from build123d import *

# Parameters (mm, degrees)
F1_DEPTH = 15
F2_DEPTH = 83.82


with BuildPart() as f1:
    # F0 (on Top) → F1 (new body, symmetric)
    with BuildSketch(Plane.XY):
        Polygon((20.593876, 37.709061), (-42.857531, 35.482697), (-40.909462, 15.167112), (-40.909462, -7.65313), (-11.131826, -49.954068), (28.386155, -49.954068), (38.404796, -35.482697), (0.953089, -31.724066), (0, -19.619845), (35.34355, -16.836887), (32.003999, 0), (13.142763, 16.280918), (28.107863, 25.464052), align=None)
    extrude(amount=F1_DEPTH, both=True)

    # F1_face (on face) → F2 (join)
    with BuildSketch(Plane(origin=(-4.856756, -2.869367, 15), x_dir=(1, 0, 0), z_dir=(0, 0, 1))):
        Polygon((5.809844, -28.854699), (4.856756, -16.750478), (40.200306, -13.96752), (36.860755, 2.869367), (17.999519, 19.150285), (32.964619, 28.333419), (25.450632, 40.578428), (-38.000776, 38.352064), (-36.052706, 18.036479), (-36.052706, -4.783763), (-6.27507, -47.084701), (33.242911, -47.084701), (43.261552, -32.61333), align=None)
    extrude(amount=F2_DEPTH)


solid = f1.part
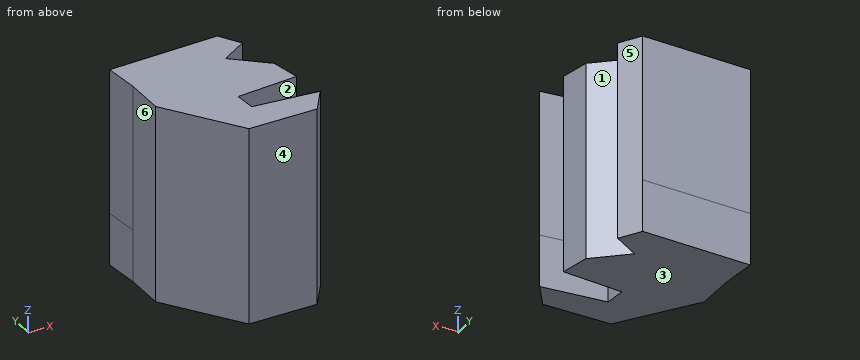
The listing builds one solid part. Answer for the finished solid, in the listing's coordinates (mm). Face numbers are marked on the shaded views. A direction names the side the tool comes from. Coordinates: 2 decimals unless noted, no trailing zeros. Order: outer loops, then holes, each group sorted by start corner. A loop starts at its lowest first (then second) coordinate and runs counter-clockwise, first axis right, second up.
Q1. A cutting plane is placed at D-D, the plane x = -38. Write down the section's boundary in (y, z).
Q2. A cutting plane is placed at A-A, the plane x = 3. Write down the section's boundary in (y, z), and give its area (3 significant figures).
Q3. A cutting plane is placed at B-B, the plane z = 90. Write down the section's boundary in (x, y).
Q4. Consider line 1 (Y direction, x = 15, z = 34); line 2 (Y direction, x = 14, z = 5.5); line 3 (Y direction, x = 12.5, z = 60.5). Determine where each line is inside the solid, lowest interval first.
Q5. For a pull along Y with two mould halves and no side action, classify the marked faces 1, 2, 3 and 4 as pulls with the +Y half, pulls with the -Y half, needs draft (parallel to the pull), parting line crosses it, or undercut.
Q6. Which of the six approach directions +Z, -Z, +X, -X, +Y, -Y give full straight-line access (tool end or side, diameter ignored) to the marked faces 5 and 6?
Q7. Given P1, Ø2, axis at y = -22, z = 61.5, coming from the -X side; P2, Ø5, axis at y = 23, z = 34.5, coming from the +X side; P3, Ø18.5, axis at y = 3, z = 62, coming from the -X side, each flat-ended and moving along its own axis, determine where each tip first touches the part or whether it passes through.
Answers follow:
1. outline: (-11.79, -15) - (35.65, -15) - (35.65, 98.82) - (-11.79, 98.82) - close
2. outline: (-49.95, -15) - (-31.93, -15) - (-31.93, 98.82) - (-49.95, 98.82) - close; (-19.38, -15) - (37.09, -15) - (37.09, 98.82) - (-19.38, 98.82) - close
2. area: 8,480 mm2
3. outline: (-42.86, 35.48) - (-40.91, 15.17) - (-40.91, -7.65) - (-11.13, -49.95) - (28.39, -49.95) - (38.4, -35.48) - (0.95, -31.72) - (0, -19.62) - (35.34, -16.84) - (32, 0) - (13.14, 16.28) - (28.11, 25.46) - (20.59, 37.71) - close
4. line 1: y = -49.95 to -33.13, -18.44 to 14.68, 17.42 to 37.51
4. line 2: y = -49.95 to -33.03, -18.52 to 15.54, 16.81 to 37.48
4. line 3: y = -49.95 to -32.88, -18.64 to 37.43
5. face 1: undercut
5. face 2: undercut
5. face 3: needs draft
5. face 4: pulls with the -Y half
6. face 5: +Z, -Z, +X, +Y
6. face 6: +Z, -Z, -X, -Y
7. P1: stops at x = -31.51
7. P2: stops at x = 28.11
7. P3: stops at x = -40.91
